Can you work these out from the model? Positions are in its coordinate system, mm. Give positions to 0.01 mm unless a question says otherwise; leave off trailing zeros. Order: outer loops, then holes, each group sorted by start corner. A loop starts at its lowest first (then second) coordinate and runs counter-clockwise, first axis right, second up.
```python
from build123d import *

# Parameters (mm, degrees)
PROFILE_EXTRUDE_DEPTH = 34
HOLES_SKETCH_R        = 5
HOLES_SKETCH_R_2      = 15
HOLES_CUT_DEPTH       = 34


with BuildPart() as part:
    # Profile Sketch → Profile Extrude (new body)
    with BuildSketch(Plane(origin=(0, 0, 0), x_dir=(0, 0, -1), z_dir=(1, 0, 0))):
        with BuildLine():
            Line((-199, 19.974984355), (0.5, 9.987492178))
            ThreePointArc((0.5, 9.987492178), (10, 0), (0.5, -9.987492178))
            Line((0.5, -9.987492178), (-199, -19.974984355))
            ThreePointArc((-199, -19.974984355), (-220, 0), (-199, 19.974984355))
        make_face()
    extrude(amount=PROFILE_EXTRUDE_DEPTH)

    # Holes Sketch → Holes Cut (cut)
    with BuildSketch(Plane(origin=(34, 0, 0), x_dir=(0, 0, -1), z_dir=(1, 0, 0))):
        Circle(HOLES_SKETCH_R)
        with Locations((-200, 0)):
            Circle(HOLES_SKETCH_R_2)
    extrude(amount=-HOLES_CUT_DEPTH, mode=Mode.SUBTRACT)


solid = part.part
```
1) Suppose I cut it at A-A (y = 0). Please give me the cut outline in (x, z), and give its area (3 significant figures).
2) Suppose I cut it at C-C (z = 172). Please give me the cut outline in (x, y).
3) Suppose I cut it at B-B (x = 15). Please give me the cut outline in (y, z), and give its area (3 significant figures).
4) If I drill on line 1 (Y direction, x = 21, z = 200); line 2 (Z direction, x = 22, y = 1); line 3 (Z direction, x = 12, y = 4), over which ranges is the centre line in solid material (lowest first)?
5) We'd pull the mould along Z, two halves only. Please class faces 1 (the face through (16.76, -14.91, 97.85)), 2 (the face through (17.238, 0.66, 214.985)), 3 (the face through (34, 0, 103)): +Z half, -Z half, draft (parallel to the pull), parting line (faces both ways), or undercut.
6) I'm going to push flat-ended pins straight in: pin 1 Ø12 at (x, z) = (6.5, 87.5) entering from +Y; pin 2 Ø1.5 at (x, z) = (21.5, 22.5) entering from +Y; pin 3 Ø3 at (x, z) = (11.5, 184.5) entering from +Y. Where does each tip first touch, or does it pass through?
7) Suppose I cut it at D-D (z = 29). Please give me the cut outline in (x, y), and give its area (3 significant figures).
Results:
1. outline: (0, -10) - (34, -10) - (34, -5) - (0, -5) - close; (0, 5) - (34, 5) - (34, 185) - (0, 185) - close; (0, 215) - (34, 215) - (34, 220) - (0, 220) - close
1. area: 6,460 mm2
2. outline: (0, -18.62) - (34, -18.62) - (34, 18.62) - (0, 18.62) - close
3. outline: (-19.97, 199) - (-9.99, -0.5) arc R10 ccw to (9.99, -0.5) - (19.97, 199) arc R20 ccw (long way) to start; hole circle Ø30 at (0, 200); hole circle Ø10 at (0, 0)
3. area: 6,010 mm2
4. line 1: y = -20 to -15, 15 to 20
4. line 2: z = -9.95 to -4.9, 4.9 to 185.03, 214.97 to 219.97
4. line 3: z = -9.17 to -3, 3 to 185.54, 214.46 to 219.6
5. face 1: -Z half
5. face 2: undercut
5. face 3: draft
6. pin 1: stops at y = 14.69
6. pin 2: stops at y = 11.18
6. pin 3: stops at y = 19.32
7. outline: (0, -11.46) - (34, -11.46) - (34, 11.46) - (0, 11.46) - close
7. area: 780 mm2
